Input: part model. Units: mm. Frame: model coordinates. A direction names the side the tool comes from. Coordinates: 2 decimals unless noted, no trailing zeros. Order: outer loops, then holes, each group sorted by start corner. A loop starts at its lowest first (then second) coordinate and runs counter-clockwise, first axis right, second up. Notation, with made-up numbers: M 76,34.5 L 122,34.5 A14 cw 122,40.5 Z; hole C 54,42 d10. An arc over 180 degrees is marked long. One line per item, written item: value.
```python
from build123d import *

# Parameters (mm, degrees)
F0_R       = 103.556034567
F1_DEPTH   = 88.646
F1_FACE_R  = 103.556034567
F1_FACE1_R = 103.556034567
F3_DEPTH   = 28.448
F3_TAPER   = -3
F4_DEPTH   = 18.034


# Not quite as in the source:
# - a feature names something its author has since deleted; it is built from what else it names


with BuildPart() as f1:
    # F0 (on Front) → F1 (new body)
    with BuildSketch(Plane.XZ):
        Circle(F0_R)
    extrude(amount=F1_DEPTH)

    # F1_face (on face) + F1_face1 (on face) → F3 (join)
    with BuildSketch(Plane.XZ.offset(88.646)):
        Circle(F1_FACE_R)
    with BuildSketch(Plane(origin=(0, 0, 0), x_dir=(1, 0, 0), z_dir=(0, 1, 0))):
        Circle(F1_FACE1_R)
    extrude(amount=F3_DEPTH, taper=F3_TAPER, dir=(0, -1, 0))

    # F4 (add): a face of the model
    f4_faces = [f1.faces().sort_by_distance(p)[0] for p in [
        (0, -117.094, 0),
    ]]
    extrude(f4_faces, amount=-F4_DEPTH)


solid = f1.part
```
(1) Cut plane B-B on y = -8. Output: boundary loops of the cut face in (x, z), plus the area to 3 significant figures.
Data:
outline: C 0,0 d207.95
area: 34,000 mm2
(2) Access query for faces 1 (the flat face through (77, -28.448, 70)), 2 (the flat face through (-1, 0, 1)). Directions: +Z, -Z, +X, -X, +Y, -Y. A direction counts if a zero-diameter tool reaches every point of the face in a straight line with its end or side. Return the directions, or none.
Data:
face 1: none
face 2: +Z, -Z, +X, -X, +Y
(3) First-contact query: pin 1 (2 mm diameter, centred on y = -31.5, z = -60, fed in from +X); pin 2 (4 mm diameter, centred on y = -96.5, z = -75.5, fed in from +X); pin 3 (8 mm diameter, centred on y = -100.5, z = -27, fed in from -X); pin 4 (6 mm diameter, centred on x = -54, z = 31, fed in from +Y). Flat tips, straight axial feed; report the tip coordinate or a pass-through.
Data:
pin 1: stops at x = 85.1
pin 2: stops at x = 73.54
pin 3: stops at x = -102.5
pin 4: stops at y = 0
(4) Ray query, line 1 (Z direction, x = 2, y = -102); line 2 (X direction, y = -106, z = 49.5); line 3 (X direction, y = -19, z = -1). Return the intervals inside material, ascending. Write a range as from..to.
Data:
line 1: z = -105.03..105.03
line 2: x = -92.65..92.65
line 3: x = -104.55..104.55
(5) Draft query along Y for faces 3 (the conical face through (-22.54, -8.1, 101.51)), 4 (the flat face through (-1, -117.094, 1)), 5 (the conical face through (-103.49, -89.3, 4.55)). Return one class per face: released by +Y, released by -Y, zero draft, split by the parting line, or undercut.
Data:
face 3: released by +Y
face 4: released by -Y
face 5: undercut
(6) Cut plane A-A on y = -46.5. Output: boundary loops of the cut face in (x, z).
Data:
outline: C 0,0 d207.11
